from build123d import *

# Parameters (mm, degrees)
F0_W     = 120
F0_H     = 10
F1_DEPTH = 100
F3_DEPTH = 100.001
F5_DEPTH = 100.001
F6_W     = 10
F6_H     = 10
F7_DEPTH = 70.001


with BuildPart() as f1:
    # F0 (on Right) → F1 (new body)
    with BuildSketch(Plane.YZ):
        with Locations((0, 5)):
            Rectangle(F0_W, F0_H)
        with BuildLine():
            Line((-60, 10), (60, 10))
            ThreePointArc((60, 10), (0, 70), (-60, 10))
        make_face()
    extrude(amount=F1_DEPTH)

    # F2 (on face) → F3 (cut, through all)
    with BuildSketch(Plane.YZ.offset(100)):
        with BuildLine():
            ThreePointArc((40, 10), (0, 50), (-40, 10))
            Line((-40, 10), (40, 10))
        make_face()
    extrude(amount=-F3_DEPTH, mode=Mode.SUBTRACT)

    # F4 (on face) → F5 (cut, through all)
    with BuildSketch(Plane.YZ.offset(100)):
        with BuildLine():
            ThreePointArc((-5, 10), (0, 5), (5, 10))
            Line((5, 10), (-5, 10))
        make_face()
        with BuildLine():
            Line((-5, 10), (5, 10))
            ThreePointArc((5, 10), (0, 15), (-5, 10))
        make_face()
        with BuildLine():
            ThreePointArc((39.6875, 14.990225), (36.355655, 13.423266), (35, 10))
            Line((35, 10), (40, 10))
            ThreePointArc((40, 10), (39.921799, 12.5), (39.6875, 14.990225))
        make_face()
        with BuildLine():
            Line((-40, 10), (-35, 10))
            ThreePointArc((-35, 10), (-36.355655, 13.423266), (-39.6875, 14.990225))
            ThreePointArc((-39.6875, 14.990225), (-39.921799, 12.5), (-40, 10))
        make_face()
        with BuildLine():
            ThreePointArc((-39.6875, 14.990225), (-43.644345, 6.576734), (-35, 10))
            Line((-35, 10), (-40, 10))
            ThreePointArc((-40, 10), (-39.921799, 12.5), (-39.6875, 14.990225))
        make_face()
        with BuildLine():
            Line((40, 10), (35, 10))
            ThreePointArc((35, 10), (40, 5), (45, 10))
            ThreePointArc((45, 10), (43.423266, 13.644345), (39.6875, 14.990225))
            ThreePointArc((39.6875, 14.990225), (39.921799, 12.5), (40, 10))
        make_face()
    extrude(amount=-F5_DEPTH, mode=Mode.SUBTRACT)

    # F6 (on face) → F7 (cut, through all)
    with BuildSketch(Plane(origin=(0, 0, 0), x_dir=(1, 0, 0), z_dir=(0, 0, -1))):
        with Locations((50, 40)):
            Rectangle(F6_W, F6_H)
        with Locations((50, 0)):
            Rectangle(F6_W, F6_H)
        with Locations((50, -40)):
            Rectangle(F6_W, F6_H)
    extrude(amount=-F7_DEPTH, mode=Mode.SUBTRACT)


solid = f1.part
Source: CAD feature listing. Evaluate the final solid. Frame: model axes, mm. A direction names the side the tool comes from. Round coordinates to 2 decimals unless told otherwise and drop trailing zeros. Loops run counter-clockwise (first coordinate to the right, second up) from the corner with the lowest first, then second, coordinate; pieces in that order, holes last. Notation, with made-up numbers: M 15,-17 L 35,-17 A35 cw 35,19 Z; hole C -35,63 d8. An arc over 180 degrees is marked long. Return JSON: item names as keys, results as strings. Group by question number.
1. Reachability of faces 4 (the face through (49, -60, 5)), 5 (the face through (45, 40, 34)), 6 (the face through (51, -20, 10)) from +Z, -Z, +X, -X, +Y, -Y: full face, straight path, thin tool, end or side. Return the list, or none.
2. Pin query (flat end, axial travel): pin 1 (5 mm diameter, centred on x = 50.5, z = 47.5, fed in from +Y); pin 2 (8 mm diameter, centred on x = 58, z = 42.5, fed in from +Y); pin 3 (9 mm diameter, centred on x = 60.5, y = 24, fed in from +Z). Return the tip coordinate at first contact, or that it passes through.
3. Mould query, pull axis X, two halves, no side actions, for faces 1 (the face through (50, 5, 60)), 2 (the face through (100, -1, 51)), 3 (the face through (49, 60, 5)). Classes: released by +X, released by -X, zero draft, split by the parting line, or undercut.
4. Section query C-C on z = 46. Output: boundary loops of the cut face in (x, y), and give its area (3 significant figures).
5. Section query A-A on y = 0. Output: boundary loops of the cut face in (x, z), and give its area (3 significant figures).
6. Section query D-D on y = 29.5. Output: boundary loops of the cut face in (x, z).
7. Material intervals for line 1 along X through (y, z) = (40, 49); line 2 along Y through (x, z) = (48.5, 4); line 3 along Z through (x, y) = (61, -17), sorted ascending. Write a range as from..to.
8. Section query B-B on x = 32. Output: boundary loops of the cut face in (y, z), and give its area (3 significant figures).
Checks:
{
 "1": {"face 4": "+Z, -Z, +X, -X, -Y", "face 5": "+Z, -Z", "face 6": "+X, -X"},
 "2": {"pin 1": "stops at y = 48.73", "pin 2": "stops at y = 52.8", "pin 3": "stops at z = 66.74"},
 "3": {"face 1": "undercut", "face 2": "released by +X", "face 3": "zero draft"},
 "4": {"outline": "M 0,-48 L 100,-48 L 100,-17.44 L 0,-17.44 Z; M 0,17.44 L 100,17.44 L 100,48 L 0,48 Z; hole M 45,-45 L 55,-45 L 55,-35 L 45,-35 Z; hole M 45,35 L 55,35 L 55,45 L 45,45 Z", "area": "5,910 mm²"},
 "5": {"outline": "M 0,0 L 45,0 L 45,5 L 0,5 Z; M 0,50 L 45,50 L 45,70 L 0,70 Z; M 55,0 L 100,0 L 100,5 L 55,5 Z; M 55,50 L 100,50 L 100,70 L 55,70 Z", "area": "2,250 mm²"},
 "6": {"outline": "M 0,0 L 100,0 L 100,10 L 0,10 Z; M 0,37.01 L 100,37.01 L 100,62.25 L 0,62.25 Z"},
 "7": {"line 1": "x = 0..45, 55..100", "line 2": "y = -60..-45, -35..-5, 5..35, 45..60", "line 3": "z = 0..10, 46.21..67.54"},
 "8": {"outline": "M -60,0 L 60,0 L 60,10 A60 ccw -60,10 Z; hole M -39.69,14.99 A5 ccw long -35,10 L -5,10 A5 ccw 5,10 L 35,10 A5 ccw long 39.69,14.99 A40 ccw Z", "area": "4,180 mm²"}
}
